Input: part model. Units: mm. Frame: model coordinates. Give positions to 0.01 mm unless a question says otherwise; leave off trailing zeros. Loops run counter-clockwise (first coordinate to the right, second up) from the corner with the lowest first, then second, coordinate; pieces in that order, holes last.
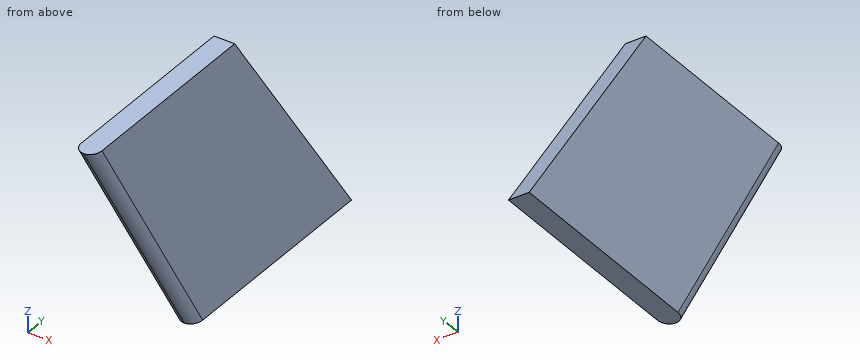
from build123d import *

# Parameters (mm, degrees)
F1_DEPTH = 10
F2_R     = 4.99999


# Not quite as in the source:
# - a fillet or chamfer is up to 0.001 mm smaller than in the source, because OpenCascade refuses the exact size


with BuildPart() as f1:
    # F0 (on Right) → F1 (new body)
    with BuildSketch(Plane.YZ):
        Polygon((0, 120), (0, 0), (111.5350200628, 0), (28.5433451417, 120), align=None)
        Polygon((-71.4566548583, 120), (0, 0), (0, 120), align=None)
    extrude(amount=F1_DEPTH)

    # F2 (radius 5 in the source; OpenCascade refuses exactly that, so slightly less here)
    f2_edges = [f1.edges().sort_by_distance(p)[0] for p in [
        (0, -35.728327, 60),
        (10, -35.728327, 60),
    ]]
    fillet(f2_edges, radius=F2_R)


solid = f1.part
(1) Cut plane A-A (y = 52). Return the cut outline in (x, z), and give its area (3 significant figures).
Values follow:
outline: (0, 0) - (10, 0) - (10, 86.08) - (0, 86.08) - close
area: 861 mm2
(2) Pin query (flat end, axial travel): pin 1 Ø4 at (x, z) = (7, 101.5) entering from -Y; pin 2 Ø1 at (x, z) = (6.5, 23.5) entering from +Y. Return the tip coordinate at first contact, or that it passes through.
Values follow:
pin 1: stops at y = -61.36
pin 2: stops at y = 95.63
(3) Cut plane B-B (x = 7.75). Return the cut outline in (y, z), and give its area (3 significant figures).
Values follow:
outline: (-70.5, 120) - (0.96, 0) - (111.54, 0) - (28.54, 120) - close
area: 12,600 mm2
(4) Ray query, probe 1 along Y at (x, z) = (6, 114); probe 2 along Z at (x, y) = (3.25, 94); probe 3 along Z at (x, y) = (1.25, 34.5). Return the intervals inside material, ascending.
Values follow:
probe 1: y = -67.77 to 32.69
probe 2: z = 0 to 25.35
probe 3: z = 0 to 111.39
